For this review, take the finished solid that the model builds, in its own axes (mm). Coordinates: 2 decimals unless noted, no trailing zeros. Loops run counter-clockwise (first coordinate to the right, second up) from the corner with the lowest first, then second, coordinate; pieces in that order, holes last. Notation, with made-up numbers: (-10.75, 5) -> (26.25, 5) arc R33 ccw to (26.25, 38) -> close; hole circle Ø7 at (49.5, 34.5). An arc over 180 degrees is marked (long way). Use a Markdown table: item, result.
from build123d import *

# Parameters (mm, degrees)
SKETCH1_R                      = 30.1625
SKETCH1_R_2                    = 26.9875
BOSS_EXTRUDE1_DEPTH            = 76.2
BOSS_EXTRUDE1_DEPTH_BACK       = 76.2
CUT_EXTRUDE1_REACH             = 32.163
SKETCH2_R                      = 4.318
CUT_EXTRUDE1_DIRECTION_2_REACH = 32.163


with BuildPart() as part:
    # Sketch1 → Boss-Extrude1 (new body, two sides)
    with BuildSketch(Plane(origin=(0, 0, 0), x_dir=(1, 0, 0), z_dir=(0, 1, 0))) as boss_extrude1_sk:
        Circle(SKETCH1_R)
        Circle(SKETCH1_R_2, mode=Mode.SUBTRACT)
    extrude(amount=BOSS_EXTRUDE1_DEPTH)
    extrude(boss_extrude1_sk.sketch, amount=-BOSS_EXTRUDE1_DEPTH_BACK)

    # Sketch2 → Cut-Extrude1 (cut, up to next)
    with BuildSketch(Plane.XY, mode=Mode.PRIVATE) as cut_extrude1_sk1:
        with Locations((0, 63.5)):
            Circle(SKETCH2_R)
    cut_extrude1_tool1 = extrude(cut_extrude1_sk1.sketch, amount=-CUT_EXTRUDE1_REACH, mode=Mode.PRIVATE) & part.part
    add(cut_extrude1_tool1.solids().sort_by_distance((0, 63.5, 0))[0], mode=Mode.SUBTRACT)
    # Sketch2 → Cut-Extrude1 (cut, up to next)
    with BuildSketch(Plane.XY, mode=Mode.PRIVATE) as cut_extrude1_sk2:
        with Locations((0, -63.5)):
            Circle(SKETCH2_R)
    cut_extrude1_tool2 = extrude(cut_extrude1_sk2.sketch, amount=-CUT_EXTRUDE1_REACH, mode=Mode.PRIVATE) & part.part
    add(cut_extrude1_tool2.solids().sort_by_distance((0, -63.5, 0))[0], mode=Mode.SUBTRACT)

    # Sketch2 → Cut-Extrude1 direction 2 (cut, up to next)
    with BuildSketch(Plane.XY, mode=Mode.PRIVATE) as cut_extrude1_direction_2_sk1:
        with Locations((0, 63.5)):
            Circle(SKETCH2_R)
    cut_extrude1_direction_2_tool1 = extrude(cut_extrude1_direction_2_sk1.sketch, amount=CUT_EXTRUDE1_DIRECTION_2_REACH, mode=Mode.PRIVATE) & part.part
    add(cut_extrude1_direction_2_tool1.solids().sort_by_distance((0, 63.5, 0))[0], mode=Mode.SUBTRACT)
    # Sketch2 → Cut-Extrude1 direction 2 (cut, up to next)
    with BuildSketch(Plane.XY, mode=Mode.PRIVATE) as cut_extrude1_direction_2_sk2:
        with Locations((0, -63.5)):
            Circle(SKETCH2_R)
    cut_extrude1_direction_2_tool2 = extrude(cut_extrude1_direction_2_sk2.sketch, amount=CUT_EXTRUDE1_DIRECTION_2_REACH, mode=Mode.PRIVATE) & part.part
    add(cut_extrude1_direction_2_tool2.solids().sort_by_distance((0, -63.5, 0))[0], mode=Mode.SUBTRACT)


solid = part.part
(1) Take a section at A-A on z = 0. Write out the cut boundary in (x, y).
Found:
| item | result |
|---|---|
| outline | (-30.16, -76.2) -> (-26.99, -76.2) -> (-26.99, 76.2) -> (-30.16, 76.2) -> close; (26.99, -76.2) -> (30.16, -76.2) -> (30.16, 76.2) -> (26.99, 76.2) -> close |
(2) Take a section at D-D on y = 28.5. Write out the cut boundary in (x, z) (1 decimal), plus the area to 3 significant figures.
Found:
| item | result |
|---|---|
| outline | circle Ø60.3 at (0, 0); hole circle Ø54 at (0, 0) |
| area | 570 mm^2 |
(3) Mouldability with a two-part tool opening along X and no side actions: class faces 1 (the face through (-30.133, 1.067, -1.326)), 2 (the face through (-4.314, -63.31, 28.377)), 3 (the face through (-22.5, 76.2, 15.5)) as pulls with the +X half, pulls with the -X half, needs draft (parallel to the pull), parting line crosses it, or undercut.
Found:
| item | result |
|---|---|
| face 1 | parting line crosses it |
| face 2 | undercut |
| face 3 | needs draft |
(4) Take a section at B-B on x = 0. Write out the cut boundary in (y, z), plus the area to 3 significant figures.
Found:
| item | result |
|---|---|
| outline | (-76.2, -30.16) -> (-67.82, -30.16) -> (-67.82, -26.99) -> (-76.2, -26.99) -> close; (-76.2, 26.99) -> (-67.82, 26.99) -> (-67.82, 30.16) -> (-76.2, 30.16) -> close; (-59.18, -30.16) -> (59.18, -30.16) -> (59.18, -26.99) -> (-59.18, -26.99) -> close; (-59.18, 26.99) -> (59.18, 26.99) -> (59.18, 30.16) -> (-59.18, 30.16) -> close; (67.82, -30.16) -> (76.2, -30.16) -> (76.2, -26.99) -> (67.82, -26.99) -> close; (67.82, 26.99) -> (76.2, 26.99) -> (76.2, 30.16) -> (67.82, 30.16) -> close |
| area | 858 mm^2 |
(5) For pin 1 Ø12 at (y, z) = (-14.5, -9) entering from +X; pin 2 Ø3 at (x, y) = (-5.5, -10) entering from -Z; pin 3 Ø10 at (y, z) = (41, 16) entering from -X, all flat-tipped, find the tip position at first contact; note any pin that passes through.
Found:
| item | result |
|---|---|
| pin 1 | stops at x = 30.01 |
| pin 2 | stops at z = -29.9 |
| pin 3 | stops at x = -28.09 |
(6) For line 1 along Y through (x, z) = (0, -28.1); line 2 along X through (y, z) = (-15.5, 0), list the stretches that pass through material, from the lowest coordinate up.
Found:
| item | result |
|---|---|
| line 1 | y = -76.2 to -67.82, -59.18 to 59.18, 67.82 to 76.2 |
| line 2 | x = -30.16 to -26.99, 26.99 to 30.16 |
